Design review of the part built by this model. Coordinates are the model's own, in mm. Coordinates: 2 decimals unless noted, no trailing zeros. Write each loop counter-clockwise with the first axis right and the second up, starting at its lowest first coordinate (ties: lowest second). Pieces come first, ordered by that corner, then holes.
```python
from build123d import *

# Parameters (mm, degrees)
BOSS_EXTRUDE3_DEPTH = 33
SKETCH3_W           = 10.19694267
SKETCH3_H           = 11
CUT_EXTRUDE1_DEPTH  = 10
SKETCH4_W           = 3.453847424
SKETCH4_H           = 11.5
SKETCH4_W_2         = 5
SKETCH4_W_3         = 11.907694848
CUT_EXTRUDE2_DEPTH  = 10.007450565


with BuildPart() as part:
    # Sketch1 → Boss-Extrude3 (new body)
    with BuildSketch(Plane(origin=(0, 0, 0), x_dir=(1, 0, 0), z_dir=(0, 1, 0))):
        with BuildLine():
            Line((-97.485150278, 1.701609628), (-102.484388754, 1.78887166))
            ThreePointArc((-102.484388754, 1.78887166), (-72.478445072, -72.478445072), (1.78887166, -102.484388754))
            Line((1.78887166, -102.484388754), (1.701609628, -97.485150278))
            ThreePointArc((1.701609628, -97.485150278), (-68.942911166, -68.942911166), (-97.485150278, 1.701609628))
        make_face()
    extrude(amount=BOSS_EXTRUDE3_DEPTH)

    # Sketch3 → Cut-Extrude1 (cut)
    with BuildSketch(Plane(origin=(0, 0, 0), x_dir=(-0.017452406437284955, 0, -0.9998476951563913), z_dir=(0.9998476951563912, 0, -0.01745240643728495))):
        with Locations((-100, 16.5)):
            Rectangle(SKETCH3_W, SKETCH3_H)
    extrude(amount=-CUT_EXTRUDE1_DEPTH, mode=Mode.SUBTRACT)

    # Sketch4 → Cut-Extrude2 (cut)
    with BuildSketch(Plane(origin=(0, 0, 0), x_dir=(-0.9998476951563914, 0, -0.01745240643727919), z_dir=(0.01745240643727919, 0, -0.9998476951563914))):
        with Locations((104.226923712, 5.75)):
            Rectangle(SKETCH4_W, SKETCH4_H)
        with Locations((95.773076288, 5.75)):
            Rectangle(SKETCH4_W, SKETCH4_H)
        with Locations((100, 5.75)):
            Rectangle(SKETCH4_W_2, SKETCH4_H)
        with Locations((100, 27.25)):
            Rectangle(SKETCH4_W_3, SKETCH4_H)
    extrude(amount=-CUT_EXTRUDE2_DEPTH, mode=Mode.SUBTRACT)


solid = part.part
```
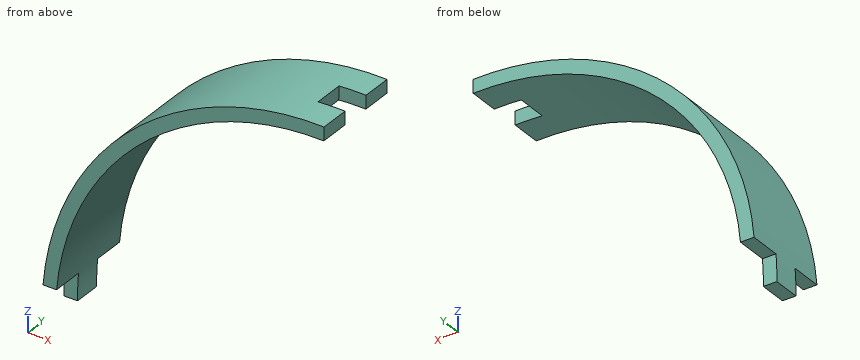
(1) Wall thickness on line 1 (X direction, y = 25.5, z = 32); line 2 (Z direction, x = -59.5, y = 8.5); line 3 (Z direction, x = -76.5, y = 29.5): over which ranges is each line inside the solid? List them lowest first.
(2) Consider section A-A (y = 17.5). Give the boundary of the cut face in (x, z), plus the area to 3 significant figures.
(3) Consider section B-B (x = -95.5). Give the boundary of the cut face in (y, z), plus the area to 3 significant figures.
(4) Insertion check: pin 1 Ø10 at (x, y) = (-42, 29) entering from -Z; pin 2 Ø12 at (x, z) = (-85.5, 12.5) entering from -Y; pin 3 Ø8 at (y, z) = (9.5, 64) entering from -X; pin 4 Ø12 at (x, y) = (-36, 20) entering from -Z. Each pin has a flat end and moves straight along its axis. Give the tip position at first contact, or say it passes through.
Results:
1. line 1: x = -97.38 to -92.1
1. line 2: z = 77.24 to 83.46
1. line 3: z = 60.45 to 68.22
2. outline: (-102.48, -1.79) - (-97.49, -1.7) arc R97.5 cw to (-8.31, 97.15) - (-8.22, 102.17) arc R102.5 ccw to start
2. area: 753 mm2
3. outline: (0, 19.65) - (33, 19.65) - (33, 37.23) - (0, 37.23) - close
3. area: 580 mm2
4. pin 1: stops at z = 85.42
4. pin 2: passes through
4. pin 3: stops at x = -83.1
4. pin 4: stops at z = 87.99
